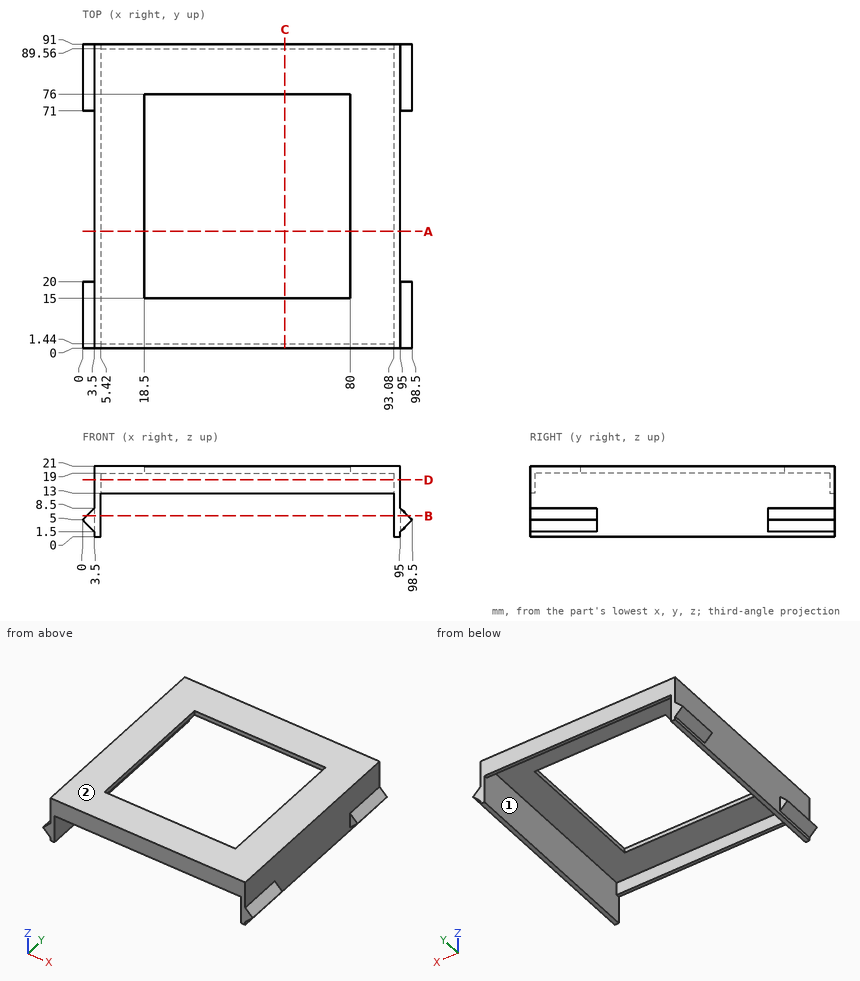
The drawing under review shows one solid part. Ordinate dimensions are in mm from its lowest x, y, z. Coordinates: 2 decimals unless noted, no trailing zeros. Order: outer loops, then holes, each group sorted by start corner. A loop starts at its lowest first (then second) coordinate and runs counter-clockwise, first axis right, second up. Notation, with made-up numbers: M 41,-37 L 93,-37 A3 cw 93,-32 Z; hole C 1,55.25 d4. An arc over 180 degrees is marked long. Use a Markdown table: item, result.
(1) Add section A-A (y = 35). Give the boundary of the cut face in (x, z), then the cut area to 3 significant figures.
Worked answers:
| item | result |
|---|---|
| outline | M 3.5,0 L 5.42,0 L 5.42,19 L 18.5,19 L 18.5,21 L 3.5,21 Z; M 80,19 L 93.08,19 L 93.08,0 L 95,0 L 95,21 L 80,21 Z |
| area | 133 mm2 |
(2) For P1, Ø5, axis at x = 51, z = 16.5, coming from the -Y side; P2, Ø0.7, axis at x = 65.5, y = 1, coming from the -Z side; P3, Ø2, axis at y = 9.5, z = 10.5, coming from the +X side; P4, Ø6, axis at y = 76.5, z = 9.5, coming from the -X side, all flat-tipped, find the tip position at first contact; note any pin that passes through.
Worked answers:
| item | result |
|---|---|
| P1 | stops at y = 0 |
| P2 | stops at z = 13 |
| P3 | stops at x = 95 |
| P4 | stops at x = 1.5 |
(3) Add section B-B (z = 6.25). Give the boundary of the cut face in (x, y), then the cut area to 3 significant figures.
Worked answers:
| item | result |
|---|---|
| outline | M 1.25,0 L 5.42,0 L 5.42,91 L 1.25,91 L 1.25,71 L 3.5,71 L 3.5,20 L 1.25,20 Z; M 93.08,0 L 97.25,0 L 97.25,20 L 95,20 L 95,71 L 97.25,71 L 97.25,91 L 93.08,91 Z |
| area | 529 mm2 |
(4) Add section D-D (z = 17). Give the boundary of the cut face in (x, y), then the cut area to 3 significant figures.
Worked answers:
| item | result |
|---|---|
| outline | M 3.5,0 L 95,0 L 95,91 L 3.5,91 Z; hole M 5.42,1.44 L 93.08,1.44 L 93.08,89.56 L 5.42,89.56 Z |
| area | 602 mm2 |
(5) Add section C-C (x = 60.5). Give the boundary of the cut face in (y, z).
Worked answers:
| item | result |
|---|---|
| outline | M 0,13 L 1.44,13 L 1.44,19 L 15,19 L 15,21 L 0,21 Z; M 76,19 L 89.56,19 L 89.56,13 L 91,13 L 91,21 L 76,21 Z |
(6) Draft analysis for pull direction Y (two halves, no side actions). For the marked faces 1 and 2, state which applies: released by +Y, released by -Y, zero draft, split by the parting line, or undercut.
Worked answers:
| item | result |
|---|---|
| face 1 | undercut |
| face 2 | zero draft |
(7) Wall thickness on probe 1 along X at (y, z) = (21.5, 16.5); probe 2 along Y at (x, z) = (62, 19.25); probe 3 along Y at (x, z) = (57.5, 13.25): over which ranges is each line inside the solid? List them lowest first.
Worked answers:
| item | result |
|---|---|
| probe 1 | x = 3.5 to 5.42, 93.08 to 95 |
| probe 2 | y = 0 to 15, 76 to 91 |
| probe 3 | y = 0 to 1.44, 89.56 to 91 |
